Design review of the part shown in the three views and the two pictorial views. Dimensions are in mm from the part's minimum x, y and z. A direction names the side the tool comes from. Coordinates: 2 decimals unless noted, no trailing zeros. Write each loop counter-clockwise with the first axis right and the second up, starting at its lowest first coordinate (ties: lowest second). Pieces come first, ordered by that corner, then holes. Notation, with made-up numbers: M 3.25,-24.5 L 11.25,-24.5 A22 cw 11.25,-7.5 Z; hole C 30.25,78 d11. An arc over 180 degrees is marked long. Answer as a JSON object with one key per item and string values.
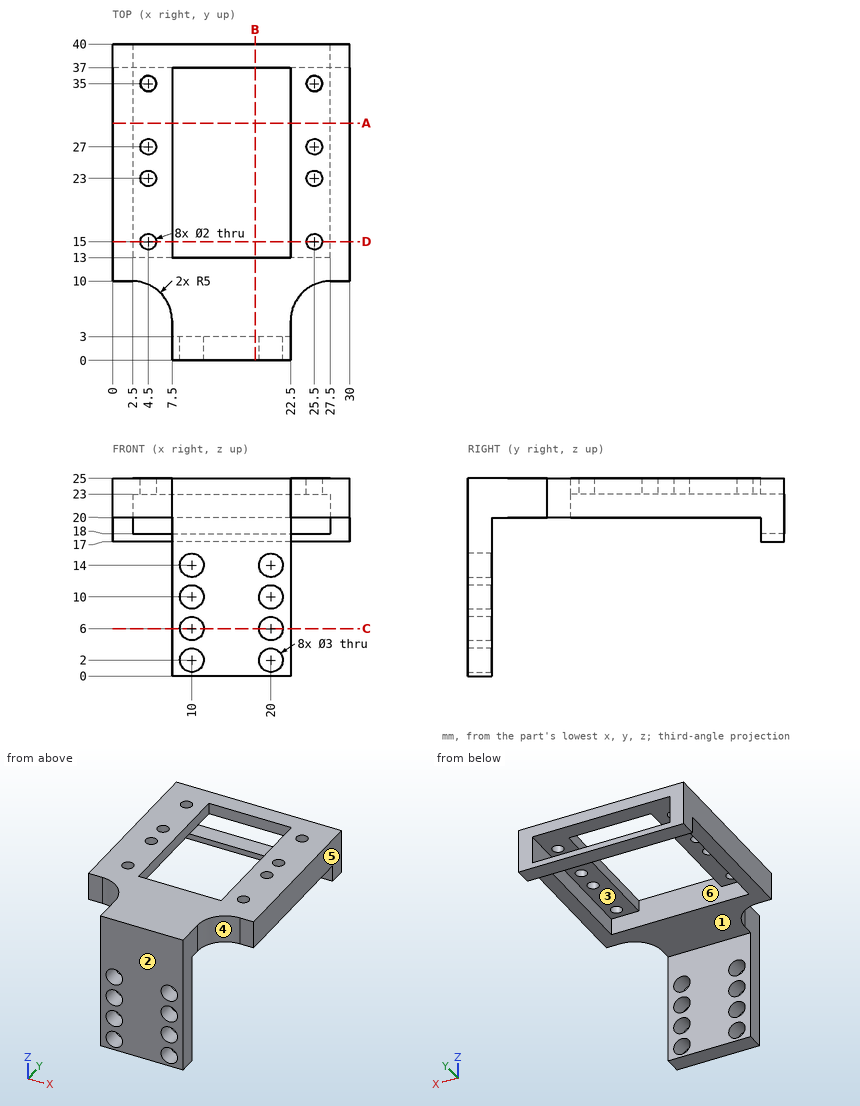
(1) Add section D-D on y = 15. Give the boundary of the cut face in (x, z), and give its area (3 significant figures).
Results list:
{"outline": "M 0,20 L 2.5,20 L 2.5,23 L 3.5,23 L 3.5,25 L 0,25 Z; M 5.5,23 L 7.5,23 L 7.5,25 L 5.5,25 Z; M 22.5,23 L 24.5,23 L 24.5,25 L 22.5,25 Z; M 26.5,23 L 27.5,23 L 27.5,20 L 30,20 L 30,25 L 26.5,25 Z", "area": "37.0 mm²"}
(2) Add section B-B on x = 18. Give the boundary of the cut face in (y, z).
Results list:
{"outline": "M 0,0 L 3,0 L 3,20 L 13,20 L 13,25 L 0,25 Z; M 37,17 L 40,17 L 40,18 L 37,18 Z; M 37,23 L 40,23 L 40,25 L 37,25 Z"}
(3) Wall thickness on line 1 along X through (y, z) = (1.7, 2); line 2 along X through (y, z) = (35, 24.2); line 3 along Y through (x, z) = (4.5, 23.45): over which ranges is each line inside the solid? List them lowest first. Write a range as from..to.
Results list:
{"line 1": "7.5..8.5, 11.5..18.5, 21.5..22.5", "line 2": "0..3.5, 5.5..7.5, 22.5..24.5, 26.5..30", "line 3": "9.58..14, 16..22, 24..26, 28..34, 36..40"}
(4) Add section C-C on z = 6. Give the boundary of the cut face in (x, y).
Results list:
{"outline": "M 7.5,0 L 8.5,0 L 8.5,3 L 7.5,3 Z; M 11.5,0 L 18.5,0 L 18.5,3 L 11.5,3 Z; M 21.5,0 L 22.5,0 L 22.5,3 L 21.5,3 Z"}
(5) Add section A-A on y = 30. Give the boundary of the cut face in (x, z).
Results list:
{"outline": "M 0,20 L 2.5,20 L 2.5,23 L 7.5,23 L 7.5,25 L 0,25 Z; M 22.5,23 L 27.5,23 L 27.5,20 L 30,20 L 30,25 L 22.5,25 Z"}
(6) Draft analysis for pull direction Y (two halves, no side actions). For the marked faces 4, 5 and 6, state which applies: released by +Y, released by -Y, zero draft, split by the parting line, or undercut.
Results list:
{"face 4": "released by -Y", "face 5": "zero draft", "face 6": "undercut"}
(7) For the marked faces 1, 2 and 3, list the 3-axis set-ups (+Z, -Z, +X, -X, +Y, -Y) from which the entire face can be reached by the end or side of a thin tool; tool diameter is ignored.
Results list:
{"face 1": "-Z, +X, -X", "face 2": "+Z, -Z, +X, -X, -Y", "face 3": "+Y"}
(8) For pin 1 Ø3 at (x, y) = (25.5, 23) entering from -Z; pin 2 Ø3 at (x, z) = (29, 23) entering from -Y; pin 3 Ø1.6 at (y, z) = (23, 24.5) entering from -X; pin 4 Ø2 at (x, y) = (15.5, 13) entering from -Z, all flat-tipped, find the tip position at first contact; note any pin that passes through.
Results list:
{"pin 1": "z = 23", "pin 2": "y = 10", "pin 3": "x = 0", "pin 4": "z = 20"}
